Check sheet for the modelled part. Datum: model origin and axes. Units: mm. A direction names the side the tool comes from. Round coordinates to 2 decimals unless told otherwise and drop trailing zeros. Loops run counter-clockwise (first coordinate to the right, second up) from the corner with the lowest first, then second, coordinate; pieces in that order, holes last. Notation, with made-up numbers: (37.25, 35.5) -> (68.25, 35.5) arc R27 cw to (68.25, 71.5) -> close; hole circle Ø4 at (59, -3.75). An arc over 180 degrees is marked (long way). Return JSON: item names as keys, results as strings.
from build123d import *

# Parameters (mm, degrees)
SKETCH_W        = 102
SKETCH_H        = 44
SKETCH_R        = 1.25
PAD_DEPTH       = 3
SKETCH001_R     = 5.5
POCKET_DEPTH    = 3.001
SKETCH002_R     = 1.5
POCKET001_DEPTH = 3.001
POCKET002_DEPTH = 3.001
FILLET_R        = 2


with BuildPart() as part:
    # Sketch → Pad (new body)
    with BuildSketch(Plane.XZ):
        with Locations((51, 22)):
            Rectangle(SKETCH_W, SKETCH_H)
        with Locations((5, 22)):
            Circle(SKETCH_R, mode=Mode.SUBTRACT)
        with Locations((97, 22)):
            Circle(SKETCH_R, mode=Mode.SUBTRACT)
    extrude(amount=PAD_DEPTH)

    # Sketch001 (on Face8 of Pad) → Pocket (cut, through all)
    with BuildSketch(Plane.XZ.offset(3)):
        with Locations((15, 30)):
            Circle(SKETCH001_R)
        with Locations((87, 30)):
            Circle(SKETCH001_R)
    extrude(amount=-POCKET_DEPTH, mode=Mode.SUBTRACT)

    # Sketch002 (on Face5 of Pocket) → Pocket001 (cut, through all)
    with BuildSketch(Plane.XZ.offset(3)):
        with Locations((39, 38)):
            Circle(SKETCH002_R)
        with Locations((63, 38)):
            Circle(SKETCH002_R)
        with Locations((39, 14)):
            Circle(SKETCH002_R)
        with Locations((63, 14)):
            Circle(SKETCH002_R)
    extrude(amount=-POCKET001_DEPTH, mode=Mode.SUBTRACT)

    # Sketch003 (on Face5 of Pocket001) → Pocket002 (cut, through all)
    with BuildSketch(Plane.XZ.offset(3)):
        with BuildLine():
            Line((50, 39.96424), (50, 32.928203))
            ThreePointArc((50, 32.928203), (44.937661, 29.499721), (44.500239, 23.401325))
            Line((38.406893, 19.88333), (44.500239, 23.401325))
            ThreePointArc((50, 39.96424), (38.875484, 32.999723), (38.406893, 19.88333))
        make_face()
        with BuildLine():
            Line((39.406972, 18.151325), (45.500399, 21.669367))
            ThreePointArc((45.500399, 21.669367), (51.000645, 19), (56.500399, 21.670379))
            Line((56.500399, 21.670379), (62.593745, 18.152384))
            ThreePointArc((39.406972, 18.151325), (51.00064, 12), (62.593745, 18.152384))
        make_face()
        with BuildLine():
            Line((57.500239, 23.402522), (63.593666, 19.884481))
            ThreePointArc((63.593666, 19.884481), (63.124196, 33.000277), (52, 39.96424))
            Line((52, 32.928203), (52, 39.96424))
            ThreePointArc((57.500239, 23.402522), (57.062017, 29.500279), (52, 32.928203))
        make_face()
    extrude(amount=-POCKET002_DEPTH, mode=Mode.SUBTRACT)

    # Fillet
    fillet_edges = [part.edges().sort_by_distance(p)[0] for p in [
        (44.500239, -1.5, 23.401325),
        (50, -1.5, 32.928203),
        (63.593666, -1.5, 19.884481),
        (56.500399, -1.5, 21.670379),
        (52, -1.5, 39.96424),
        (39.406972, -1.5, 18.151325),
        (62.593745, -1.5, 18.152384),
        (45.500399, -1.5, 21.669367),
        (50, -1.5, 39.96424),
        (38.406893, -1.5, 19.88333),
        (52, -1.5, 32.928203),
        (57.500239, -1.5, 23.402522),
    ]]
    fillet(fillet_edges, radius=FILLET_R)


solid = part.part
Q1. Section check B-B (z = 31). Record the boundary of the cut face in (x, y).
Results list:
{"outline": "(0, -3) -> (9.59, -3) -> (9.59, 0) -> (0, 0) -> close; (20.41, -3) -> (37.92, -3) -> (37.92, 0) -> (20.41, 0) -> close; (46.1, -3) -> (55.9, -3) -> (55.9, 0) -> (46.1, 0) -> close; (64.08, -3) -> (81.59, -3) -> (81.59, 0) -> (64.08, 0) -> close; (92.41, -3) -> (102, -3) -> (102, 0) -> (92.41, 0) -> close"}
Q2. Section check D-D (z = 14). Record the boundary of the cut face in (x, y), then the cut area to 3 significant figures.
Results list:
{"outline": "(0, -3) -> (37.5, -3) -> (37.5, 0) -> (0, 0) -> close; (40.5, -3) -> (43.79, -3) -> (43.79, 0) -> (40.5, 0) -> close; (58.21, -3) -> (61.5, -3) -> (61.5, 0) -> (58.21, 0) -> close; (64.5, -3) -> (102, -3) -> (102, 0) -> (64.5, 0) -> close", "area": "245 mm^2"}
Q3. Tool access check on faces 3 (the flat face through (41.78, -1.52, 21.83)), 4 (the flat face through (50, -1, 44)). Record the directions out of +Z, -Z, +X, -X, +Y, -Y that give a thin tool (end or side, any length) a straight path to the whole face; none if there is none.
Results list:
{"face 3": "+Y, -Y", "face 4": "+Z, +X, -X, +Y, -Y"}
Q4. Material ranges on line 1 (Z direction, x = 46, y = -0.3); line 2 (Z direction, x = 39, y = -1.3); line 3 (Z direction, x = 62.5, y = -2.05), recorded low to high.
Results list:
{"line 1": "0 to 12.92, 20.97 to 30.9, 39.08 to 44", "line 2": "0 to 12.5, 15.5 to 20.84, 33.21 to 36.5, 39.5 to 44", "line 3": "0 to 12.59, 15.41 to 20.79, 33.98 to 36.59, 39.41 to 44"}
Q5. Go/stop test with a flat-tipped pin: pin 1 (3.5 mm diameter, centred on x = 63, z = 38, fed in from -Y). Record where the tip stops, or that it passes through.
Results list:
{"pin 1": "y = -3"}
Q6. Draft check along X on faces 1 (the flat face through (50, -3, 22)), 2 (the cylindrical face through (40.453, -1.479, 17.837)). Enter one of: released by +X, released by -X, zero draft, split by the parting line, or undercut.
Results list:
{"face 1": "zero draft", "face 2": "undercut"}
Q7. Section check A-A (x = 87). Record the boundary of the cut face in (y, z).
Results list:
{"outline": "(-3, 0) -> (0, 0) -> (0, 24.5) -> (-3, 24.5) -> close; (-3, 35.5) -> (0, 35.5) -> (0, 44) -> (-3, 44) -> close"}
Q8. Section check C-C (x = 5). Record the boundary of the cut face in (y, z), then the cut area to 4 significant figures.
Results list:
{"outline": "(-3, 0) -> (0, 0) -> (0, 20.75) -> (-3, 20.75) -> close; (-3, 23.25) -> (0, 23.25) -> (0, 44) -> (-3, 44) -> close", "area": "124.5 mm^2"}
